Geometry check sheet. Reference: the model listing, model coordinates, mm. Face numbers are marked on the shaded views. A direction names the side the tool comes from. Coordinates: 2 decimals unless noted, no trailing zeros. Loops run counter-clockwise (first coordinate to the right, second up) from the corner with the lowest first, then second, coordinate; pieces in that order, holes last.
from build123d import *

# Parameters (mm, degrees)
SKETCH1_W           = 80
SKETCH1_H           = 29
BOSS_EXTRUDE1_DEPTH = 51.5
SKETCH2_W           = 25
SKETCH2_H           = 49.5
CUT_EXTRUDE1_DEPTH  = 100.464817901
FILLET6_R           = 2
SKETCH3_R           = 1.5
SKETCH3_R_2         = 4
CUT_EXTRUDE2_DEPTH  = 43.5
SKETCH4_R           = 4
SKETCH4_R_2         = 1.5
SKETCH4_R_3         = 2
CUT_EXTRUDE3_DEPTH  = 43.5
FILLET7_R           = 4


with BuildPart() as part:
    # Sketch1 → Boss-Extrude1 (new body)
    with BuildSketch(Plane(origin=(0, 0, 0), x_dir=(1, 0, 0), z_dir=(0, 1, 0))):
        with Locations((0, -14.5)):
            Rectangle(SKETCH1_W, SKETCH1_H)
    extrude(amount=BOSS_EXTRUDE1_DEPTH)

    # Sketch2 → Cut-Extrude1 (cut, through all)
    with BuildSketch(Plane(origin=(40, 0, 0), x_dir=(0, 0, -1), z_dir=(1, 0, 0))):
        with Locations((-14.5, 26.75)):
            Rectangle(SKETCH2_W, SKETCH2_H)
    extrude(amount=-CUT_EXTRUDE1_DEPTH, mode=Mode.SUBTRACT)

    # Fillet6
    fillet6_edges = [part.edges().sort_by_distance(p)[0] for p in [
        (0, 0, 0),
        (0, 0, 29),
    ]]
    fillet(fillet6_edges, radius=FILLET6_R)

    # Sketch3 → Cut-Extrude2 (cut)
    with BuildSketch(Plane(origin=(0, 2, 0), x_dir=(1, 0, 0), z_dir=(0, 1, 0))):
        with Locations(Location((35.5, -14.5, 0), (0, 0, 270))):
            Circle(SKETCH3_R)
        with Locations(Location((29, -14.5, 0), (0, 0, 270))):
            Circle(SKETCH3_R_2)
        with Locations(Location((22.5, -14.5, 0), (0, 0, 270))):
            Circle(SKETCH3_R)
        with Locations(Location((29, -8, 0), (0, 0, 270))):
            Circle(SKETCH3_R)
        with Locations(Location((29, -21, 0), (0, 0, 270))):
            Circle(SKETCH3_R)
        with Locations(Location((-29, -21, 0), (0, 0, 90))):
            Circle(SKETCH3_R)
        with Locations(Location((-35.5, -14.5, 0), (0, 0, 90))):
            Circle(SKETCH3_R)
        with Locations(Location((-22.5, -14.5, 0), (0, 0, 90))):
            Circle(SKETCH3_R)
        with Locations(Location((-29, -14.5, 0), (0, 0, 90))):
            Circle(SKETCH3_R_2)
        with Locations(Location((-29, -8, 0), (0, 0, 90))):
            Circle(SKETCH3_R)
        with Locations(Location((0, -14.5, 0), (0, 0, 270))):
            Circle(SKETCH3_R_2)
        with Locations(Location((6.5, -14.5, 0), (0, 0, 270))):
            Circle(SKETCH3_R)
        with Locations(Location((-6.5, -14.5, 0), (0, 0, 270))):
            Circle(SKETCH3_R)
        with Locations(Location((0, -8, 0), (0, 0, 270))):
            Circle(SKETCH3_R)
        with Locations(Location((0, -21, 0), (0, 0, 270))):
            Circle(SKETCH3_R)
    extrude(amount=-CUT_EXTRUDE2_DEPTH, mode=Mode.SUBTRACT)

    # Sketch4 → Cut-Extrude3 (cut)
    with BuildSketch(Plane.XY.offset(29)):
        with Locations((22, 40.5)):
            Circle(SKETCH4_R)
        with Locations((15.5, 40.5)):
            Circle(SKETCH4_R_2)
        with Locations((28.5, 40.5)):
            Circle(SKETCH4_R_2)
        with Locations((22, 47)):
            Circle(SKETCH4_R_2)
        with Locations((21.823366501, 34)):
            Circle(SKETCH4_R_2)
        with Locations((-21.823366501, 34)):
            Circle(SKETCH4_R_2)
        with Locations((-28.5, 40.5)):
            Circle(SKETCH4_R_2)
        with Locations((-22, 47)):
            Circle(SKETCH4_R_2)
        with Locations((-22, 40.5)):
            Circle(SKETCH4_R)
        with Locations((-15.5, 40.5)):
            Circle(SKETCH4_R_2)
        with Locations((0, 40.5)):
            Circle(SKETCH4_R)
        with Locations((6.5, 40.5)):
            Circle(SKETCH4_R_2)
        with Locations((-6.5, 40.5)):
            Circle(SKETCH4_R_2)
        with Locations((0, 47)):
            Circle(SKETCH4_R_2)
        with Locations((0, 34)):
            Circle(SKETCH4_R_2)
        with Locations((12, 43.5)):
            Circle(SKETCH4_R_2)
        with Locations((-12, 43.5)):
            Circle(SKETCH4_R_2)
        with Locations((11.68, 38.5)):
            Circle(SKETCH4_R_3)
        with Locations((11.68, 28.5)):
            Circle(SKETCH4_R_3)
        with Locations((-33.68, 38.5)):
            Circle(SKETCH4_R_3)
        with Locations((-33.68, 28.5)):
            Circle(SKETCH4_R_3)
    extrude(amount=-CUT_EXTRUDE3_DEPTH, mode=Mode.SUBTRACT)

    # Fillet7
    fillet7_edges = [part.edges().sort_by_distance(p)[0] for p in [
        (40, 51.5, 28),
        (-40, 51.5, 28),
        (40, 51.5, 1),
        (-40, 51.5, 1),
    ]]
    fillet(fillet7_edges, radius=FILLET7_R)


solid = part.part
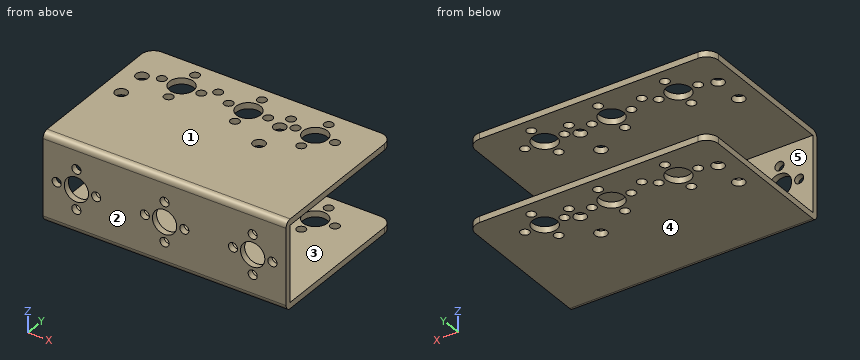
1) Mould release check, pull along Z, two halves, no side actions. Record for the marked faces 1, 2 and 3: +Z half, -Z half, draft (parallel to the pull), parting line (faces both ways), or undercut.
Data:
face 1: +Z half
face 2: draft
face 3: undercut
2) Section check D-D on x = -3. Record the cut outline in (y, z).
Data:
outline: (0, 2) arc R2 ccw to (2, 0) - (37.85, 0) - (37.85, 2) - (2, 2) - (2, 11.85) - (0, 11.85) - close; (0, 17.15) - (2, 17.15) - (2, 27) - (37.85, 27) - (37.85, 29) - (2, 29) arc R2 ccw to (0, 27) - close; (43.15, 0) - (51.5, 0) - (51.5, 2) - (43.15, 2) - close; (43.15, 27) - (51.5, 27) - (51.5, 29) - (43.15, 29) - close
3) Material ranges on probe 1 along Z at (x, y) = (-25, 28); probe 2 along X at (y, z) = (1.5, 21); probe 3 along Y at (x, z) = (22, 1.55), recorded low to high.
Data:
probe 1: z = 0 to 2, 27 to 29
probe 2: x = -40 to -30.5, -27.5 to -1.5, 1.5 to 27.5, 30.5 to 40
probe 3: y = 0.05 to 32.51, 35.49 to 36.5, 44.5 to 45.5, 48.5 to 51.5
4) Section check C-C on y = 8. Record the cut outline in (x, z).
Data:
outline: (-40, 0) - (40, 0) - (40, 2) - (-40, 2) - close; (-40, 27) - (40, 27) - (40, 29) - (-40, 29) - close
5) Depth check by flat-ended pin: pin 1 (4 mm diameter, centred on x = -23, y = 39.5, fed in from -Z); pin 2 (3.5 mm diameter, centred on x = 22.5, z = 14.5, fed in from +Y). Enter the tip coordinate at first touch or a pass-through.
Data:
pin 1: passes through
pin 2: stops at y = 2
6) Access from +Z, -Z, +X, -X, +Y, -Y to the whole of each face (thin tool, end or side, straight path). Record for the marked faces 4 and 5.
Data:
face 4: -Z, +X, -X, +Y, -Y
face 5: +X, -X, +Y
7) Section check B-B on z = 21. Record the cut outline in (x, y).
Data:
outline: (-40, 0) - (-30.5, 0) - (-30.5, 2) - (-40, 2) - close; (-27.5, 0) - (-1.5, 0) - (-1.5, 2) - (-27.5, 2) - close; (1.5, 0) - (27.5, 0) - (27.5, 2) - (1.5, 2) - close; (30.5, 0) - (40, 0) - (40, 2) - (30.5, 2) - close
8) Section check A-A on x = 15.5. Record the cut outline in (y, z).
Data:
outline: (0, 2) arc R2 ccw to (2, 0) - (39, 0) - (39, 2) - (2, 2) - (2, 27) - (39, 27) - (39, 29) - (2, 29) arc R2 ccw to (0, 27) - close; (42, 0) - (51.5, 0) - (51.5, 2) - (42, 2) - close; (42, 27) - (51.5, 27) - (51.5, 29) - (42, 29) - close
